Read the model definition and answer for the solid it produces. Units are mm, in the model's axes. A direction names the side the tool comes from. Coordinates: 2 decimals unless noted, no trailing zeros. Order: outer loops, then holes, each group sorted by start corner. A loop starts at its lowest first (then second) coordinate and runs counter-clockwise, first axis right, second up. Notation, with made-up numbers: (85, -32.5) -> (97, -32.5) arc R8 cw to (97, -24.5) -> close; hole circle Ø3 at (73, -26.75). An arc over 180 degrees is marked (long way). Answer in a Markdown table with one row per item.
Autodesk Inventor part; units mm, degrees
ref_plane "Work Plane1" through (-10.5, 3.25, -10.5) normal (0, 1, 0) x (0, 0, 1)
ref_plane "YZ Plane" through (0, 0, 0) normal (1, 0, 0) x (0, 1, 0)
ref_plane "XZ Plane" through (0, 0, 0) normal (0, 1, 0) x (-1, 0, 0)
sketch "Sketch1" plane through (0, 0, 0) normal (0, 1, 0) x (-1, 0, 0)
  circle A0 centre (0, 0) radius 15
  line L0 (0, 0) -> (0, 15)
  line L1 (0, 15) -> (40, 15)
  line L2 (40, 15) -> (40, -15)
  line L3 (40, -15) -> (0, -15)
  line L4 (0, -15) -> (0, 15)
  dimension "d0" = 30
  dimension "d1" = 15
  dimension "d2" = 40
  dimension "d3" = 30
extrude "Extrusion1" add sketch "Sketch1" along normal blind 8
sketch "Sketch2" plane through (-40, 0, -15) normal (-1, 0, 0) x (0, 0, 1)
  line L0 (0, 0) -> (30, 0)
  line L1 (30, 0) -> (30, 8)
  line L2 (0, 8) -> (30, 8)
  line L3 (0, 0) -> (0, 8)
  line L4 (0, 0) -> (30, 0)
  line L5 (0, 0) -> (30, 0)
  line L6 (30, 0) -> (30, 40)
  line L7 (30, 40) -> (0, 40)
  line L8 (0, 40) -> (0, 0)
  point P0 (15, 0)
  dimension "d6" = 30
  dimension "d7" = 40
extrude "Extrusion2" add sketch "Sketch2" against normal blind 5
sketch "Sketch3" plane through (-40, 40, 15) normal (0, 1, 0) x (1, 0, 0)
  line L0 (0, 0) -> (0, 30)
  line L1 (0, 0) -> (5, 0)
  line L2 (5, 30) -> (5, 0)
  line L3 (0, 30) -> (5, 30)
  line L4 (3, 18) -> (3, 12)
  line L5 (3, 12) -> (-3, 12)
  line L6 (-3, 12) -> (-3, 18)
  line L7 (-3, 18) -> (3, 18)
  line L8 (0, 30) -> (0, 0)
  line L9 (3, 18) -> (-3, 12) construction
  line L10 (3, 12) -> (-3, 18) construction
  point P0 (40, 15)
  point P1 (0, 15)
  dimension "d10" = 6
  dimension "d11" = 6
extrude "Extrusion3" cut sketch "Sketch3" against normal up to surface (40 mm away) contours L5 L6 L7 L0 | L0 L7 L4 L5
sketch "Sketch4" plane through (0, 0, 0) normal (0, -1, 0) x (1, 0, 0)
  circle A0 centre (0, 0) radius 5.35
  dimension "d14" = 10.7
extrude "Extrusion4" cut sketch "Sketch4" against normal blind 8
sketch "Sketch5" plane through (0, 0, 0) normal (0, -1, 0) x (1, 0, 0)
  circle A0 centre (0, 0) radius 5.35
  line L0 (-37, -3) -> (-40, -3)
  line L1 (-40, -15) -> (-40, -3)
  line L2 (0, -15) -> (-40, -15)
  arc A1 (0, -15) -> (0, 15) centre (0, 0) ccw
  line L3 (-40, 15) -> (0, 15)
  line L4 (-40, 3) -> (-40, 15)
  line L5 (-40, 3) -> (-37, 3)
  line L6 (-37, 3) -> (-37, -3)
  line L7 (-40, -15) -> (-20, -15)
  line L8 (-20, -15) -> (-20, -8)
  line L9 (-20, -8) -> (-40, -8)
  line L10 (-40, -8) -> (-40, -15)
  line L11 (-40, 15) -> (0, 15)
  line L12 (-40, 15) -> (-20, 15)
  line L13 (-20, 15) -> (-20, 8)
  line L14 (-20, 8) -> (-40, 8)
  line L15 (-40, 8) -> (-40, 15)
  line L16 (-20, -8) -> (-13, -8)
  line L17 (-13, -8) -> (-13, -15)
  line L18 (-13, -15) -> (-20, -15)
  line L19 (-20, -15) -> (-20, -8)
  line L20 (-20, 8) -> (-13, 8)
  line L21 (-13, 8) -> (-13, 15)
  line L22 (-13, 15) -> (-20, 15)
  line L23 (-20, 15) -> (-20, 8)
  line L24 (-13, -15) -> (-20, -8)
  line L25 (-20, 8) -> (-13, 15)
  dimension "d17" = 20
  dimension "d18" = 7
  dimension "d19" = 20
  dimension "d20" = 7
  dimension "d21" = 7
  dimension "d22" = 7
  dimension "d23" = 7
  dimension "d24" = 7
extrude "Extrusion5" cut sketch "Sketch5" against normal up to surface (40 mm away) contours L9 L8 L2 L1 | L24 L2 L8 | L4 L3 L13 L14 | L13 L3 L25
sketch "Sketch6" plane through (0, 8, 0) normal (0, 1, 0) x (1, 0, 0)
  line L0 (-20, -8) -> (-13, -15)
  line L1 (-13, -15) -> (0, -15)
  arc A0 (0, -15) -> (0, 15) centre (0, 0) ccw
  line L2 (0, 15) -> (-13, 15)
  line L3 (-13, 15) -> (-20, 8)
  line L4 (-20, 8) -> (-35, 8)
  line L5 (-35, 8) -> (-35, -8)
  line L6 (-35, -8) -> (-20, -8)
  circle A1 centre (0, 0) radius 5.35
  line L7 (-35, 8) -> (-35, -8)
  line L8 (-35, -8) -> (-30, -8)
  line L9 (-30, -8) -> (-30, 8)
  line L10 (-30, 8) -> (-35, 8)
  line L11 (-35, 8) -> (-35, -8)
  dimension "d27" = 5
  dimension "d28" = 16
extrude "Extrusion6" add sketch "Sketch6" along normal up to surface (32 mm away) contours L6 L5 L4 L9
sketch "Sketch8" plane through (-40, 0, 8) normal (0, 0, 1) x (1, 0, 0)
  line L0 (10, 8) -> (10, 40)
  line L1 (0, 40) -> (10, 40)
  line L2 (0, 0) -> (0, 40)
  line L3 (20, 0) -> (0, 0)
  line L4 (20, 0) -> (20, 8)
  line L5 (10, 8) -> (20, 8)
  line L6 (10, 8) -> (10, 40)
  line L7 (10, 8) -> (10, 23)
  line L8 (10, 23) -> (20, 8)
  point P0 (40, 0)
  dimension "d34" = 15
extrude "Extrusion8" add sketch "Sketch8" against normal up to surface (16 mm away) contours L0 L8 L5
sketch "Sketch9" plane through (-20, 0, -8) normal (0, 0, -1) x (-1, 0, 0)
  line L0 (0, 0) -> (0, 8)
  line L1 (20, 0) -> (0, 0)
  line L2 (20, 40) -> (20, 0)
  line L3 (10, 40) -> (20, 40)
  line L4 (10, 23) -> (10, 40)
  line L5 (10, 23) -> (0, 8)
  line L6 (20, 0) -> (0, 0)
  line L7 (0, 0) -> (0, 4)
  line L8 (0, 0) -> (0, 8)
  line L9 (0, 4) -> (6, 4)
  line L10 (6, 4) -> (13, 4)
  circle A0 centre (6, 4) radius 1.5
  circle A1 centre (13, 4) radius 1.5
  line L11 (13, 4) -> (13, 13)
  line L12 (13, 13) -> (10, 13)
  circle A2 centre (10, 13) radius 1.5
  point P0 (-20, 0)
  dimension "d37" = 4
  dimension "d38" = 6
  dimension "d39" = 7
  dimension "d40" = 3
  dimension "d41" = 3
  dimension "d42" = 9
  dimension "d43" = 3
  dimension "d44" = 3
extrude "Extrusion9" cut sketch "Sketch9" against normal up to surface (16 mm away) contours A0 L10 L9 | L9 L10 A0 | A1 L11 L10 | L10 L11 A1 | A2
sketch "Sketch10" plane through (0, 0, 0) normal (0, -1, 0) x (1, 0, 0)
  point P0 (0, 0)
sketch "Sketch11" plane through (0, 0, 0) normal (0, -1, 0) x (1, 0, 0)
  circle A0 centre (0, 0) radius 5.35
  line L0 (-13, 15) -> (-20, 8)
  line L1 (-20, 8) -> (-40, 8)
  line L2 (-40, 3) -> (-40, 8)
  line L3 (-40, 3) -> (-37, 3)
  line L4 (-37, 3) -> (-37, -3)
  line L5 (-37, -3) -> (-40, -3)
  line L6 (-40, -8) -> (-40, -3)
  line L7 (-40, -8) -> (-20, -8)
  line L8 (-20, -8) -> (-13, -15)
  line L9 (0, -15) -> (-13, -15)
  arc A1 (0, -15) -> (0, 15) centre (0, 0) ccw
  line L10 (-13, 15) -> (0, 15)
  line L11 (0, 0) -> (7.5, 0)
  circle A2 centre (7.5, 0) radius 1.5
  circle A3 centre (0, 7.5) radius 1.5
  circle A4 centre (-7.5, 0) radius 1.5
  circle A5 centre (0, -7.5) radius 1.5
  dimension "d47" = 7.5
  dimension "d48" = 3
  dimension "d51" = 360
extrude "Extrusion10" cut sketch "Sketch11" against normal blind 10 contours A2 | A3 | A4 | A5
sketch "Sketch12" plane through (0, 0, 0) normal (0, -1, 0) x (1, 0, 0)
  point P0 (0, 0)
sketch "Sketch13" plane through (0, 0, 0) normal (0, -1, 0) x (1, 0, 0)
  arc A0 (-2.2798, -5.55) -> (2.2798, -5.55) centre (0, -7.5) ccw
  arc A1 (-5.55, -2.2798) -> (-2.2798, -5.55) centre (0, 0) ccw
  arc A2 (-5.55, 2.2798) -> (-5.55, -2.2798) centre (-7.5, 0) ccw
  arc A3 (-2.2798, 5.55) -> (-5.55, 2.2798) centre (0, 0) ccw
  arc A4 (2.2798, 5.55) -> (-2.2798, 5.55) centre (0, 7.5) ccw
  arc A5 (5.55, 2.2798) -> (2.2798, 5.55) centre (0, 0) ccw
  arc A6 (5.55, -2.2798) -> (5.55, 2.2798) centre (7.5, 0) ccw
  arc A7 (2.2798, -5.55) -> (5.55, -2.2798) centre (0, 0) ccw
  point P0 (0, 0)
ref_plane "Work Plane1" through (-10.5, 3.25, -10.5) normal (0, 1, 0) x (0, 0, 1)
extrude "Extrusion11" cut sketch "Sketch13" against normal up to surface (3.25 mm away)
thicken "Thicken1" operation add thickness 0.3 both sides no extend neighbours yes toward (0.8094149, 0, 0.5872372) faces at (2.4282, 2.1667, -5.7383) (-4.513, 2.1667, -3.9539) (-7.296, 2.1667, -2.9931) (-4.7637, 2.1667, 3.6479) (-2.4282, 2.1667, 5.7383) (5.3877, 1.0833, 2.6405) (7.296, 2.1667, 2.9931) (4.7637, 2.1667, -3.6479)
sketch "Sketch14" plane through (0, 0, 0) normal (0, -1, 0) x (1, 0, 0)
  arc A0 (5.67, -2.7461) -> (5.67, 2.7461) centre (7.5, 0) ccw
  arc A1 (2.7461, -5.67) -> (5.67, -2.7461) centre (0, 0) ccw
  arc A2 (-2.7461, -5.67) -> (2.7461, -5.67) centre (0, -7.5) ccw
  arc A3 (-5.67, -2.7461) -> (-2.7461, -5.67) centre (0, 0) ccw
  arc A4 (-5.67, 2.7461) -> (-5.67, -2.7461) centre (-7.5, 0) ccw
  arc A5 (-2.7461, 5.67) -> (-5.67, 2.7461) centre (0, 0) ccw
  arc A6 (2.7461, 5.67) -> (-2.7461, 5.67) centre (0, 7.5) ccw
  arc A7 (5.67, 2.7461) -> (2.7461, 5.67) centre (0, 0) ccw
  line L0 (-13, 15) -> (-20, 8)
  line L1 (-20, 8) -> (-40, 8)
  line L2 (-40, 3) -> (-40, 8)
  line L3 (-40, 3) -> (-37, 3)
  line L4 (-37, 3) -> (-37, -3)
  line L5 (-37, -3) -> (-40, -3)
  line L6 (-40, -8) -> (-40, -3)
  line L7 (-40, -8) -> (-20, -8)
  line L8 (-20, -8) -> (-13, -15)
  line L9 (0, -15) -> (-13, -15)
  arc A8 (0, -15) -> (0, 15) centre (0, 0) ccw
  line L10 (-13, 15) -> (0, 15)
  line L11 (-37, 0) -> (-29.5, 0)
  circle A9 centre (-29.5, 0) radius 1.5
  line L12 (-29.5, 0) -> (-17.5, 0)
  circle A10 centre (-17.5, 0) radius 1.5
  dimension "d59" = 7.5
  dimension "d60" = 3
  dimension "d61" = 12
  dimension "d62" = 3
extrude "Extrusion12" cut sketch "Sketch14" against normal blind 10 contours A9 L12 L11 | L11 L12 A9 | A10
chamfer "Chamfer1" distance 2 angle 45 6 edges at (-6.5, 0, -15) (15, 0, 0) (-6.5, 0, 15) (15, 8, 0) (-6.5, 8, -15) (-6.5, 8, 15)
fillet "Fillet1" radius 2 4 edges at (-14, 1, -14) (-14, 7, -14) (-14, 1, 14) (-14, 7, 14)
properties part number "dog_bone_3"
Q1. The part is cut by section B-B (y = 25). Write down the section's boundary in (x, z).
Outcome:
| item | result |
|---|---|
| outline | (-40, -8) -> (-30, -8) -> (-30, 8) -> (-40, 8) -> (-40, 3) -> (-37, 3) -> (-37, -3) -> (-40, -3) -> close |
Q2. The part is cut by section C-C (x = -36). Write down the section's boundary in (y, z), then the cut area to 3 significant figures.
Outcome:
| item | result |
|---|---|
| outline | (0, -8) -> (40, -8) -> (40, 8) -> (0, 8) -> close |
| area | 640 mm² |
Q3. Consider line 1 (X direction, y = 33, z = 7); line 2 (Z direction, x = 4, y = 2.5); line 3 (Y direction, x = 6.5, z = 8.75). Determine where each line is inside the solid, lowest interval first.
Outcome:
| item | result |
|---|---|
| line 1 | -40 to -30 |
| line 2 | -14.46 to -4.87, 4.87 to 14.46 |
| line 3 | 0 to 8 |
Q4. For a pull along Z with two mould halves and no side action, classify faces 4 (the face through (-31.5, 4.07, -0.11)), 5 (the face through (-19, 4, 0)), 6 (the face through (-17, 4, 11)), 7 (the face through (13.122, 7.875, -0.289)) as pulls with the +Z half, pulls with the -Z half, needs draft (parallel to the pull), parting line crosses it, or undercut.
Outcome:
| item | result |
|---|---|
| face 4 | needs draft |
| face 5 | undercut |
| face 6 | pulls with the +Z half |
| face 7 | parting line crosses it |
Q5. The part is cut by section D-D (x = -22). Write down the section's boundary in (y, z).
Outcome:
| item | result |
|---|---|
| outline | (0, -8) -> (11, -8) -> (11, 8) -> (0, 8) -> close |
Q6. The part is cut by section A-A (x = -7.5). Write down the section's boundary in (y, z), then the cut area to 3 significant figures.
Outcome:
| item | result |
|---|---|
| outline | (0, -13) -> (2, -15) -> (6, -15) -> (8, -13) -> (8, -1.5) -> (3.25, -1.5) -> (3.25, -3.3) -> (0, -3.3) -> close; (0, 3.3) -> (3.25, 3.3) -> (3.25, 1.5) -> (8, 1.5) -> (8, 13) -> (6, 15) -> (2, 15) -> (0, 13) -> close |
| area | 196 mm² |
Q7. Given pin 1 (10.5 mm diameter, centred on x = 7.5, z = 0, fed in from +Y); pin 2 (5 mm diameter, centred on x = 0, z = -7.5, fed in from -Y); pin 3 (1.8 mm diameter, centred on x = 0, z = 7.5, fed in from +Y); pin 4 (16 mm diameter, centred on x = -27, y = 29, fed in from +Z), each flat-ended and moving along its own axis, determine where each tip first touches the part or whether it passes through.
Outcome:
| item | result |
|---|---|
| pin 1 | y = 8 |
| pin 2 | y = 3.25 |
| pin 3 | through |
| pin 4 | z = 8 |
Q8. For faces 1 (the face through (-7, 7, -14)), 2 (the face through (-39, 20, -3)), 3 (the face through (10.8, 1.6, -0.1)), determine the directions among +Z, -Z, +X, -X, +Y, -Y from which every point of the face is accessible in a straight line to the end or side of a thin tool.
Outcome:
| item | result |
|---|---|
| face 1 | -Z, +X, -X, +Y |
| face 2 | -X, +Y, -Y |
| face 3 | -Y |
